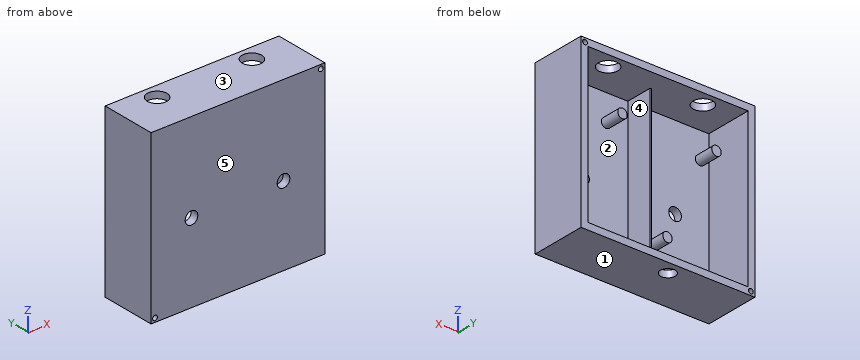
from build123d import *

# Parameters (mm, degrees)
SKETCH1_W           = 55.88
SKETCH1_H           = 54.102
BOSS_EXTRUDE1_DEPTH = 17.78
SKETCH3_W           = 51.562
SKETCH3_H           = 49.784
CUT_EXTRUDE1_DEPTH  = 15.24
SKETCH4_R           = 1.524
BOSS_EXTRUDE2_DEPTH = 6.35
SKETCH6_W           = 0.508
SKETCH6_H           = 49.784
BOSS_EXTRUDE3_DEPTH = 8.636
SKETCH7_R           = 3.175
CUT_EXTRUDE3_DEPTH  = 2.54
SKETCH8_R           = 2.38125
CUT_EXTRUDE5_DEPTH  = 2.54
SKETCH9_R           = 2.032
CUT_EXTRUDE6_DEPTH  = 2.54
SKETCH10_R          = 2.032
CUT_EXTRUDE7_DEPTH  = 2.54
SKETCH11_R          = 0.762
CUT_EXTRUDE8_DEPTH  = 49.276


with BuildPart() as part:
    # Sketch1 → Boss-Extrude1 (new body)
    with BuildSketch(Plane(origin=(0, 0, 0), x_dir=(1, 0, 0), z_dir=(0, 1, 0))):
        with Locations((27.94, 27.051)):
            Rectangle(SKETCH1_W, SKETCH1_H)
    extrude(amount=BOSS_EXTRUDE1_DEPTH)

    # Sketch3 → Cut-Extrude1 (cut)
    with BuildSketch(Plane(origin=(0, 17.78, 0), x_dir=(1, 0, 0), z_dir=(0, 1, 0))):
        with Locations((27.94, 27.051)):
            Rectangle(SKETCH3_W, SKETCH3_H)
    extrude(amount=-CUT_EXTRUDE1_DEPTH, mode=Mode.SUBTRACT)

    # Sketch4 → Boss-Extrude2 (add)
    with BuildSketch(Plane(origin=(0, 2.54, 0), x_dir=(1, 0, 0), z_dir=(0, 1, 0))):
        with Locations(Location((20.701, 40.64, 0), (0, 0, 270))):
            Circle(SKETCH4_R)
        with Locations(Location((4.953, 10.668, 0), (0, 0, 270))):
            Circle(SKETCH4_R)
        with Locations(Location((50.927, 40.767, 0), (0, 0, 270))):
            Circle(SKETCH4_R)
        with Locations(Location((35.179, 10.795, 0), (0, 0, 270))):
            Circle(SKETCH4_R)
    extrude(amount=BOSS_EXTRUDE2_DEPTH)

    # Sketch6 → Boss-Extrude3 (add)
    with BuildSketch(Plane(origin=(0, 2.54, 0), x_dir=(1, 0, 0), z_dir=(0, 1, 0))):
        with Locations((27.94, 27.051)):
            Rectangle(SKETCH6_W, SKETCH6_H)
    extrude(amount=BOSS_EXTRUDE3_DEPTH)

    # Sketch7 → Cut-Extrude3 (cut)
    with BuildSketch(Plane.XY):
        with Locations((12.7, 12.954)):
            Circle(SKETCH7_R)
        with Locations((43.18, 12.954)):
            Circle(SKETCH7_R)
    extrude(amount=-CUT_EXTRUDE3_DEPTH, mode=Mode.SUBTRACT)

    # Sketch8 → Cut-Extrude5 (cut)
    with BuildSketch(Plane(origin=(0, 0, -54.102), x_dir=(-1, 0, 0), z_dir=(0, 0, -1))):
        with Locations((-24.384, 13.462)):
            Circle(SKETCH8_R)
    extrude(amount=-CUT_EXTRUDE5_DEPTH, mode=Mode.SUBTRACT)

    # Sketch9 → Cut-Extrude6 (cut)
    with BuildSketch(Plane(origin=(0, 2.54, 0), x_dir=(1, 0, 0), z_dir=(0, 1, 0))):
        with Locations(Location((12.996559759, 28.702, 0), (0, 0, 270))):
            Circle(SKETCH9_R)
    extrude(amount=-CUT_EXTRUDE6_DEPTH, mode=Mode.SUBTRACT)

    # Sketch10 → Cut-Extrude7 (cut)
    with BuildSketch(Plane(origin=(0, 2.54, 0), x_dir=(1, 0, 0), z_dir=(0, 1, 0))):
        with Locations(Location((42.587559759, 28.702, 0), (0, 0, 270))):
            Circle(SKETCH10_R)
    extrude(amount=-CUT_EXTRUDE7_DEPTH, mode=Mode.SUBTRACT)

    # Sketch11 → Cut-Extrude8 (cut)
    with BuildSketch(Plane(origin=(0, 17.78, 0), x_dir=(1, 0, 0), z_dir=(0, 1, 0))):
        with Locations(Location((1.27, 52.832, 0), (0, 0, 270))):
            Circle(SKETCH11_R)
        with Locations(Location((54.61, 1.27, 0), (0, 0, 270))):
            Circle(SKETCH11_R)
    extrude(amount=-CUT_EXTRUDE8_DEPTH, mode=Mode.SUBTRACT)


solid = part.part
Input: part model. Units: mm. Frame: model coordinates. Face numbers are marked on the shaded views. A direction names the side the tool comes from. Give positions to 0.01 mm unless a question says otherwise; leave off trailing zeros. Write each loop counter-clockwise with the first axis right and the second up, starting at its lowest first coordinate (ties: lowest second). Pieces come first, ordered by that corner, then holes.
Q1. Set-up query: the marked faces 4 and 5. Return all of +Z, -Z, +X, -X, +Y, -Y with unobstructed straight access to the full face (end or side cutting, diameter ignored); none if empty.
Q2. Pull-direction query (Z, two-part tool) for the marked faces 1, 2 and 3; classes: pulls with the +Z half, pulls with the -Z half, needs draft (parallel to the pull), parting line crosses it, or undercut.
Q3. Section A-A, the plane x = 54.61. Output: boundary loops of the cut face in (y, z).
Q4. Section C-C, the plane y = 12.25. Output: boundary loops of the cut face in (x, z), plus the area to 3 significant figures.
Q5. Material intervals for probe 1 along X at (y, z) = (6.5, -9); probe 2 along Z at (x, y) = (18.5, 14.75); probe 3 along X at (y, z) = (16.5, -4.5), sorted ascending.
Q6. First-contact query: P1, Ø2.5, axis at x = 13, z = -28.7, coming from the -Y side; P2, Ø0.9, axis at x = 51.5, z = -41, coming from the +Y side; P3, Ø1, axis at x = 12, z = -44, coming from the +Y side. Flat tips, straight axial feed; report the tip coordinate or a pass-through.
Q7. Section B-B, the plane z = -1.27. Output: boundary loops of the cut face in (x, y) (3 decimals).
Q8. Section D-D, the plane z = -40.64. Output: boundary loops of the cut face in (x, y) (3 decimals), plus the area to 3 significant figures.
Filled in:
1. face 4: +Y
1. face 5: +Z, -Z, +X, -X, -Y
2. face 1: pulls with the -Z half
2. face 2: undercut
2. face 3: pulls with the +Z half
3. outline: (0, -54.1) - (17.78, -54.1) - (17.78, -2.03) - (0, -2.03) - close; (0, -0.51) - (17.78, -0.51) - (17.78, 0) - (0, 0) - close
4. outline: (0, -54.1) - (22.33, -54.1) - (22.33, -51.94) - (2.16, -51.94) - (2.16, -2.16) - (9.6, -2.16) - (9.6, 0) - (0, 0) - close; (15.8, -2.16) - (40.08, -2.16) - (40.08, 0) - (15.8, 0) - close; (26.43, -54.1) - (55.88, -54.1) - (55.88, 0) - (46.28, 0) - (46.28, -2.16) - (53.72, -2.16) - (53.72, -51.94) - (26.43, -51.94) - close; hole circle Ø1.52 at (1.27, -52.83); hole circle Ø1.52 at (54.61, -1.27)
4. area: 417 mm2
5. probe 1: x = 0 to 2.16, 27.69 to 28.19, 53.72 to 55.88
5. probe 2: z = -54.1 to -51.94, -2.16 to 0
5. probe 3: x = 0 to 2.16, 53.72 to 55.88
6. P1: passes through
6. P2: stops at y = 8.89
6. P3: stops at y = 2.54
7. outline: (0, 0) - (53.848, 0) - (53.848, 17.78) - (0, 17.78) - close; (55.372, 0) - (55.88, 0) - (55.88, 17.78) - (55.372, 17.78) - close; hole circle Ø6.35 at (12.7, 12.954); hole circle Ø6.35 at (43.18, 12.954)
8. outline: (0, 0) - (55.88, 0) - (55.88, 17.78) - (53.721, 17.78) - (53.721, 2.54) - (52.446, 2.54) - (52.446, 8.89) - (49.408, 8.89) - (49.408, 2.54) - (28.194, 2.54) - (28.194, 11.176) - (27.686, 11.176) - (27.686, 2.54) - (22.225, 2.54) - (22.225, 8.89) - (19.177, 8.89) - (19.177, 2.54) - (2.159, 2.54) - (2.159, 17.78) - (0, 17.78) - close
8. area: 251 mm2
